The listing builds one solid part. Answer for the finished solid, in the listing's coordinates (mm). Give positions to 0.01 mm unless a question says otherwise; leave off trailing zeros. Order: outer loops, then holes, each group sorted by start corner. A loop starts at its lowest first (then second) coordinate and runs counter-clockwise, first axis right, second up. Notation, with made-up numbers: (81, 54) - (125, 54) arc R32 cw to (125, 80) - close; hole circle Ø5 at (29.5, 11.25). An arc over 180 degrees is marked (long way). Use CSV: the item, a comma, the result in double quotes.
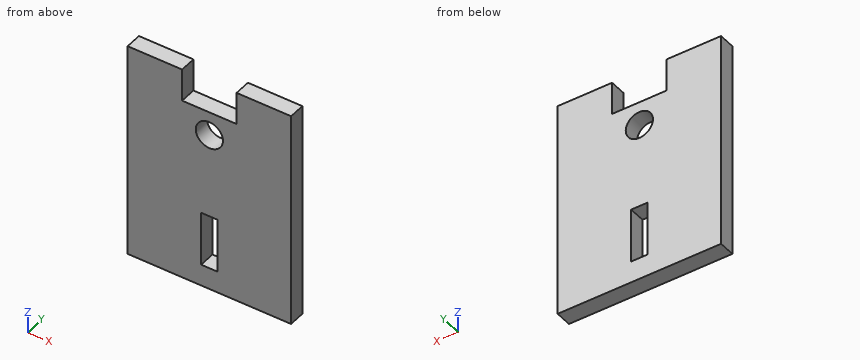
```python
from build123d import *

# Parameters (mm, degrees)
F0_W     = 3
F0_H     = 10
F0_R     = 2.5
F1_DEPTH = 3


with BuildPart() as f1:
    # F0 (on Front) → F1 (new body)
    with BuildSketch(Plane.XZ):
        Polygon((5, 4.380814), (-5, 4.380814), (-5, 10.380814), (-15, 10.380814), (-15, -29.619186), (15, -29.619186), (15, 10.380814), (5, 10.380814), align=None)
        with Locations((0, -20.619186)):
            Rectangle(F0_W, F0_H, mode=Mode.SUBTRACT)
        Circle(F0_R, mode=Mode.SUBTRACT)
    extrude(amount=F1_DEPTH)


solid = f1.part
```
Item 1: The part is cut by section B-B (x = 0). Give the vertices of the cut face in (y, z).
Taken from the geometry:
outline,"(-3, -29.62) - (0, -29.62) - (0, -25.62) - (-3, -25.62) - close; (-3, -15.62) - (0, -15.62) - (0, -2.5) - (-3, -2.5) - close; (-3, 2.5) - (0, 2.5) - (0, 4.38) - (-3, 4.38) - close"
Item 2: The part is cut by section C-C (y = -1.75). Give the vertices of the cut face in (x, z), and give its area (3 significant figures).
Taken from the geometry:
outline,"(-15, -29.62) - (15, -29.62) - (15, 10.38) - (5, 10.38) - (5, 4.38) - (-5, 4.38) - (-5, 10.38) - (-15, 10.38) - close; hole circle Ø5 at (0, 0); hole (-1.5, -25.62) - (1.5, -25.62) - (1.5, -15.62) - (-1.5, -15.62) - close"
area,"1,090 mm^2"
Item 3: The part is cut by section A-A (z = 0). Give the vertices of the cut face in (x, y).
Taken from the geometry:
outline,"(-15, -3) - (-2.5, -3) - (-2.5, 0) - (-15, 0) - close; (2.5, -3) - (15, -3) - (15, 0) - (2.5, 0) - close"
Item 4: Find the intervals of material crossed by line 1 along Z through (x, y) = (0, -1.85); line 2 along Z through (x, y) = (1, -1.2); line 3 along X through (y, z) = (-1.95, -2), in increasing order.
Taken from the geometry:
line 1,"-29.62 to -25.62, -15.62 to -2.5, 2.5 to 4.38"
line 2,"-29.62 to -25.62, -15.62 to -2.29, 2.29 to 4.38"
line 3,"-15 to -1.5, 1.5 to 15"
Item 5: The part is cut by section D-D (x = -3.5). Give the vertices of the cut face in (y, z), and give its area (3 significant figures).
Taken from the geometry:
outline,"(-3, -29.62) - (0, -29.62) - (0, 4.38) - (-3, 4.38) - close"
area,"102 mm^2"
Item 6: This flat-tipped pin is pushed along its axis until it touches: pin 1 (1.5 mm diameter, centred on x = 2.5, y = -1, fed in from +Z). Where does it stop, or does it pass through?
Taken from the geometry:
pin 1,"z = 4.38"
